Can you work these out from the model? Positions are in its coordinate system, mm. Face numbers are marked on the shaded views. A direction names the side the tool comes from. Coordinates: 2 decimals unless noted, no trailing zeros. Write each loop counter-clockwise with the first axis right and the second up, starting at its lowest first coordinate (ties: lowest second). Pieces come first, ordered by that corner, then holes. Notation, with made-up numbers: (-13, -14) - (36, -14) arc R21 cw to (36, 19) - close; hole circle Ø6 at (0.5, 24.25). An arc over 180 degrees is marked (long way). Use one line per item in the form item = value. Start each with the question number.
(1) If I drill on probe 1 along Y at (x, z) = (18.25, 5.5); probe 2 along Y at (x, z) = (9.25, 4.75); probe 3 along Y at (x, z) = (4.5, 10), over which ranges is the centre line in solid material (lowest first)? Write a range as from..to.
(2) If we section it at A-A on x = 15.5: Please give me the cut outline in (y, z), then the cut area to 3 significant figures.
(3) On a 3-axis mill with a long thin cutter (end or side, diameter ignored), from which of +Z, -Z, +X, -X, +Y, -Y can I reach the whole of each face in a straight line? I mean the marked faces 5, 6 and 7. Say none if no direction works.
(4) If we section it at D-D on y = -4: Please give me the cut outline in (x, z).
(5) If we section it at B-B on x = 13.25: Please give me the cut outline in (y, z), then the cut area to 3 significant figures.
(6) Thinking about a two-plate mould opening in Y: for the marked faces 1, 2, 3 and 4, which applies, pulls with the +Y half, pulls with the -Y half, needs draft (parallel to the pull), parting line crosses it, or undercut?
(7) For pin 1 Ø1.5 at (x, y) = (13.5, 2) entering from -Z; pin 2 Ø1.6 at (x, y) = (10, -8) entering from -Z; pin 3 Ø0.6 at (x, y) = (11.5, -7.5) entering from +Z, each with a flat end and sliding along its axis, tell me the tip position at first contact or that it passes through.
(8) If we section it at C-C on z = 6.05: Please give me the cut outline in (x, y), then the cut area to 3 significant figures.
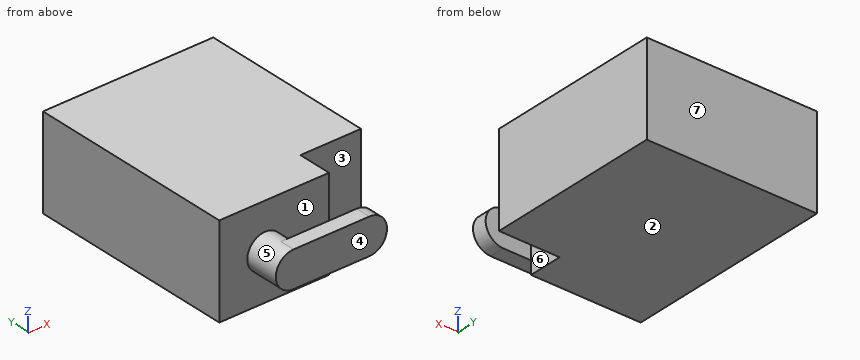
Autodesk Inventor part; units mm, degrees
ref_plane "YZ Plane" through (0, 0, 0) normal (1, 0, 0) x (0, 1, 0)
ref_plane "XZ Plane" through (0, 0, 0) normal (0, 1, 0) x (-1, 0, 0)
ref_plane "XY Plane" through (0, 0, 0) normal (0, 0, 1) x (1, 0, 0)
sketch "Sketch1" plane through (0, 0, 0) normal (0, 0, 1) x (1, 0, 0)
  line L0 (0, 0) -> (22.5, 0)
  line L1 (22.5, 0) -> (22.5, 23.3)
  line L2 (22.5, 23.3) -> (0, 23.3)
  line L3 (0, 23.3) -> (0, 0)
  line L4 (0, 0) -> (14.5, 0)
  line L5 (14.5, 0) -> (14.5, -4.5)
  line L6 (0, -4.5) -> (0, 0)
  line L7 (0, -4.5) -> (14.5, -4.5)
  dimension "d0" = 23.3
  dimension "d1" = 22.5
  dimension "d2" = 14.5
  dimension "d3" = 4.5
extrude "Extrusion1" add sketch "Sketch1" along normal blind 12.1
sketch "Sketch2" plane through (0, -4.5, 0) normal (0, -1, 0) x (1, 0, 0)
  line L0 (0, 0) -> (14.5, 0)
  line L1 (14.5, 0) -> (14.5, 12.1)
  line L2 (0, 12.1) -> (14.5, 12.1)
  line L3 (0, 0) -> (0, 12.1)
  line L4 (0, 0) -> (0, 12.1)
  line L5 (0, 6.05) -> (14.5, 6.05) construction
  line L6 (0, 12.1) -> (14.5, 12.1)
  line L7 (0, 0) -> (14.5, 0)
  circle A0 centre (6.05, 6.05) radius 6.05 construction
  line L8 (6.05, 6.05) -> (6.05, 0) construction
  circle A1 centre (6.05, 6.05) radius 2.35
  dimension "d6" = 4.7
extrude "Extrusion2" add sketch "Sketch2" along normal blind 4.5 contours A1
sketch "Sketch3" plane through (6.05, -9, 6.05) normal (0, -1, 0) x (1, 0, 0)
  line L0 (0, 0) -> (10, 0) construction
  line L1 (0, -2.35) -> (10, -2.35)
  line L2 (10, 2.35) -> (0, 2.35)
  arc A0 (0, 2.35) -> (0, -2.35) centre (0, 0) ccw
  arc A1 (10, -2.35) -> (10, 2.35) centre (10, 0) ccw
  circle A2 centre (0, 0) radius 2.35
  point P0 (-6.05, -6.05)
  point P1 (5, 0)
  point P2 (-2.35, 0)
  dimension "d9" = 10
extrude "Extrusion3" add sketch "Sketch3" against normal blind 2
properties part number "servo"
Reported:
q1.probe_1 = -9..-7, 0..23.3
q1.probe_2 = -9..-7, -4.5..23.3
q1.probe_3 = -4.5..23.3
q2.outline = (-9, 3.7) - (-7, 3.7) - (-7, 8.4) - (-9, 8.4) - close; (0, 0) - (23.3, 0) - (23.3, 12.1) - (0, 12.1) - close
q2.area = 291 mm2
q3.face_5 = none
q3.face_6 = +Z, -Z, +X
q3.face_7 = +Z, -Z, +X, -X, +Y
q4.outline = (0, 0) - (14.5, 0) - (14.5, 12.1) - (0, 12.1) - close
q5.outline = (-9, 3.7) - (-7, 3.7) - (-7, 8.4) - (-9, 8.4) - close; (-4.5, 0) - (23.3, 0) - (23.3, 12.1) - (-4.5, 12.1) - close
q5.area = 346 mm2
q6.face_1 = undercut
q6.face_2 = needs draft
q6.face_3 = undercut
q6.face_4 = pulls with the -Y half
q7.pin_1 = 0
q7.pin_2 = 3.7
q7.pin_3 = 8.4
q8.outline = (0, -4.5) - (3.7, -4.5) - (3.7, -9) - (18.4, -9) - (18.4, -7) - (8.4, -7) - (8.4, -4.5) - (14.5, -4.5) - (14.5, 0) - (22.5, 0) - (22.5, 23.3) - (0, 23.3) - close
q8.area = 631 mm2
